```python
from build123d import *
from build123d import SkipClean  # not in build123d's __all__

# Parameters (mm, degrees)
F1_DEPTH = 20
F2_R     = 16.5
F2_R_2   = 16
F3_DEPTH = 10
F4_R     = 16.5
F4_R_2   = 16
F5_DEPTH = 10


with BuildPart() as f1:
    # F0 (on Front) → F1 (new body)
    with BuildSketch(Plane.XZ):
        with BuildLine():
            Line((-3.8441673982, 15.5313353262), (-3.9642976294, 16.0166895551))
            ThreePointArc((-3.9642976294, 16.0166895551), (-7.8229406478, 14.52761507), (-11.1900395345, 12.1257171011))
            Line((-11.1900395345, 12.1257171011), (-10.8509474274, 11.7582711284))
            ThreePointArc((-10.8509474274, 11.7582711284), (-7.5858818403, 14.0873843103), (-3.8441673982, 15.5313353262))
        make_face()
    extrude(amount=F1_DEPTH)



with BuildPart() as f1b:
    # F0 (on Front) → F1, piece 2 (new body)
    with BuildSketch(Plane.XZ):
        with BuildLine():
            ThreePointArc((-15.6899392355, 3.1346142961), (-14.4174640671, 6.9380638419), (-12.2390866075, 10.3055693202))
            Line((-12.2390866075, 10.3055693202), (-12.621558064, 10.6276183614))
            ThreePointArc((-12.621558064, 10.6276183614), (-14.8680098192, 7.154878337), (-16.1802498366, 3.2325709928))
            Line((-16.1802498366, 3.2325709928), (-15.6899392355, 3.1346142961))
        make_face()
    extrude(amount=F1_DEPTH)


with BuildPart() as f1c:
    # F0 (on Front) → F1, piece 3 (new body)
    with BuildSketch(Plane.XZ):
        with BuildLine():
            Line((-15.959090724, 1.1434261073), (-16.4578123091, 1.1791581731))
            ThreePointArc((-16.4578123091, 1.1791581731), (-16.2336959024, -2.952476477), (-14.9887120925, -6.8984425639))
            Line((-14.9887120925, -6.8984425639), (-14.5345086958, -6.6893988498))
            ThreePointArc((-14.5345086958, -6.6893988498), (-15.7417657236, -2.8630074928), (-15.959090724, 1.1434261073))
        make_face()
    extrude(amount=F1_DEPTH)


with BuildPart() as f1d:
    # F0 (on Front) → F1, piece 4 (new body)
    with BuildSketch(Plane.XZ):
        with BuildLine():
            Line((-13.581495765, -8.458307915), (-14.0059175077, -8.7226300373))
            ThreePointArc((-14.0059175077, -8.7226300373), (-11.3966659743, -11.9317226195), (-8.0713200038, -14.3911011877))
            Line((-8.0713200038, -14.3911011877), (-7.8267345492, -13.9550072124))
            ThreePointArc((-7.8267345492, -13.9550072124), (-11.05131246, -11.5701552674), (-13.581495765, -8.458307915))
        make_face()
    extrude(amount=F1_DEPTH)


with BuildPart() as f1e:
    # F0 (on Front) → F1, piece 5 (new body)
    with BuildSketch(Plane.XZ):
        with BuildLine():
            Line((-6.0159922312, -14.8259177616), (-6.2039919884, -15.2892276917))
            ThreePointArc((-6.2039919884, -15.2892276917), (-2.2068058623, -16.3517585564), (1.9290419923, -16.3868482934))
            Line((1.9290419923, -16.3868482934), (1.8705861743, -15.890277133))
            ThreePointArc((1.8705861743, -15.890277133), (-2.1399329573, -15.8562507213), (-6.0159922312, -14.8259177616))
        make_face()
    extrude(amount=F1_DEPTH)


with BuildPart() as f1f:
    # F0 (on Front) → F1, piece 6 (new body)
    with BuildSketch(Plane.XZ):
        with BuildLine():
            Line((6.0190930987, 14.8246591282), (6.2071897581, 15.287929726))
            ThreePointArc((6.2071897581, 15.287929726), (2.210225959, 16.3512966217), (-1.9256144656, 16.3872514147))
            Line((-1.9256144656, 16.3872514147), (-1.8672625121, 15.8906680385))
            ThreePointArc((-1.8672625121, 15.8906680385), (2.1432494148, 15.8558027847), (6.0190930987, 14.8246591282))
        make_face()
    extrude(amount=F1_DEPTH)


with BuildPart() as f1g:
    # F0 (on Front) → F1, piece 7 (new body)
    with BuildSketch(Plane.XZ):
        with BuildLine():
            ThreePointArc((14.0077416326, 8.7197003592), (11.3991613724, 11.929338624), (8.0743298799, 14.3894126701))
            Line((8.0743298799, 14.3894126701), (7.8296532169, 13.9533698619))
            ThreePointArc((7.8296532169, 13.9533698619), (11.0537322399, 11.5678435142), (13.5832646134, 8.455467015))
            Line((13.5832646134, 8.455467015), (14.0077416326, 8.7197003592))
        make_face()
    extrude(amount=F1_DEPTH)


with BuildPart() as f1h:
    # F0 (on Front) → F1, piece 8 (new body)
    with BuildSketch(Plane.XZ):
        with BuildLine():
            ThreePointArc((16.4580585827, -1.17571582), (16.2336959024, 2.952476477), (14.9901546477, 6.8953073636))
            Line((14.9901546477, 6.8953073636), (14.5359075371, 6.6863586557))
            ThreePointArc((14.5359075371, 6.6863586557), (15.7417657236, 2.8630074928), (15.9593295347, -1.1400880679))
            Line((15.9593295347, -1.1400880679), (16.4580585827, -1.17571582))
        make_face()
    extrude(amount=F1_DEPTH)


with BuildPart() as f1i:
    # F0 (on Front) → F1, piece 9 (new body)
    with BuildSketch(Plane.XZ):
        with BuildLine():
            ThreePointArc((3.9676476045, -16.0158600296), (7.8259790826, -14.5259785005), (11.192575513, -12.1233763195))
            Line((11.192575513, -12.1233763195), (10.8534065581, -11.7560012795))
            ThreePointArc((10.8534065581, -11.7560012795), (7.5888282013, -14.0857973339), (3.8474158589, -15.5305309377))
            Line((3.8474158589, -15.5305309377), (3.9676476045, -16.0158600296))
        make_face()
    extrude(amount=F1_DEPTH)


with BuildPart() as f1j:
    # F0 (on Front) → F1, piece 10 (new body)
    with BuildSketch(Plane.XZ):
        with BuildLine():
            ThreePointArc((12.6237806679, -10.6249781952), (14.8695060132, -7.1517683773), (16.1809256095, -3.22918665))
            Line((16.1809256095, -3.22918665), (15.6905945304, -3.1313325091))
            ThreePointArc((15.6905945304, -3.1313325091), (14.4189149219, -6.9350481235), (12.2412418598, -10.303009159))
            Line((12.2412418598, -10.303009159), (12.6237806679, -10.6249781952))
        make_face()
    extrude(amount=F1_DEPTH)


with BuildPart() as f1_1:
    add(f1.part, clean=False)

    add(f1b.part)  # F3 merges F1b

    add(f1c.part)  # F3 merges F1c

    add(f1d.part)  # F3 merges F1d

    add(f1e.part)  # F3 merges F1e

    add(f1f.part)  # F3 merges F1f

    add(f1g.part)  # F3 merges F1g

    add(f1h.part)  # F3 merges F1h

    add(f1i.part)  # F3 merges F1i

    add(f1j.part)  # F3 merges F1j
    # F2 (on face) → F3 (join)
    with BuildSketch(Plane.XZ):
        Circle(F2_R)
        Circle(F2_R_2, mode=Mode.SUBTRACT)
    extrude(amount=-F3_DEPTH)

    # F4 (on face) → F5 (join)
    with BuildSketch(Plane.XZ.offset(20)):
        Circle(F4_R)
        Circle(F4_R_2, mode=Mode.SUBTRACT)
    with SkipClean():  # cleaning this boolean's faces spoils the solid; the shape is the same uncleaned
        extrude(amount=F5_DEPTH)


solid = f1_1.part
```
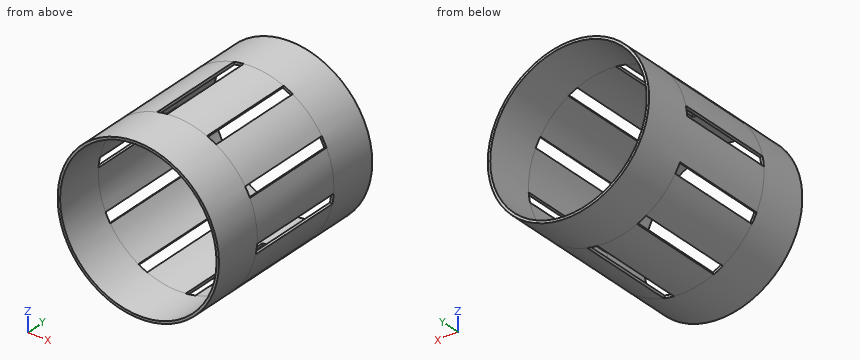
CAD build for the part. Positions are in the model's coordinates, mm. Coordinates: 2 decimals unless noted, no trailing zeros. Order: outer loops, then holes, each group sorted by start corner. A loop starts at its lowest first (then second) coordinate and runs counter-clockwise, first axis right, second up.
(1) Saw through at C-C, the plane y = -9.5. Count the separate pieces of the cut face and the enclosed holes in it, and give its area (3 significant figures).
Solution:
separate pieces: 10
enclosed holes: 0
area: 40.8 mm2
(2) Pin check, flat tips, straight feed: pin 1 Ø1.5 at (x, z) = (7.5, 15) entering from -Y; pin 2 Ø1 at (x, y) = (7, -6) entering from +Z; pin 3 Ø10 at (x, z) = (-7.5, 1.5) entering from -Y; pin 4 Ø4 at (y, z) = (-13.5, -11) entering from +X. Stop position of each tip, or through.
Solution:
pin 1: stops at y = -30
pin 2: stops at z = -14.13
pin 3: passes through
pin 4: stops at x = 13.83
(3) Saw through at B-B, the plane z = 0. Write the cut outline in (x, y).
Solution:
outline: (-16.5, -30) - (-16, -30) - (-16, 10) - (-16.5, 10) - close; (16, -30) - (16.5, -30) - (16.5, 10) - (16, 10) - close
(4) Drill centre lines: L1, parallel to X at y = -15, z = -1; L2, parallel to Z at x = 0, y = -23.5; L3, parallel to Z at x = -13.5, y = 7. Where is each one in solid material? Low to high.
Solution:
L1: x = -16.47 to -15.97, 15.97 to 16.47
L2: z = -16.5 to -16, 16 to 16.5
L3: z = -9.49 to -8.59, 8.59 to 9.49
(5) Saw through at A-A, the plane x = 0. Write the cut outline in (y, z).
Solution:
outline: (-30, -16.5) - (10, -16.5) - (10, -16) - (-30, -16) - close; (-30, 16) - (10, 16) - (10, 16.5) - (-30, 16.5) - close
